The figure shows three views and two pictorial views of one solid part (mm, origin at its lowest corner). Answer the questions. A direction names the side the tool comes from. Round coordinates to 2 decimals unless told otherwise and drop trailing zeros. Write each loop counter-clockwise with the first axis right and the second up, starting at its lowest first coordinate (ties: lowest second). Pieces come first, ordered by that corner, then holes. Notation, with made-up numbers: (21, -7) -> (44, -7) arc R33 ccw to (44, 27) -> close; hole circle Ø2 at (41.5, 71.5). An arc over 180 degrees is marked (long way). One line per item, written item: value.
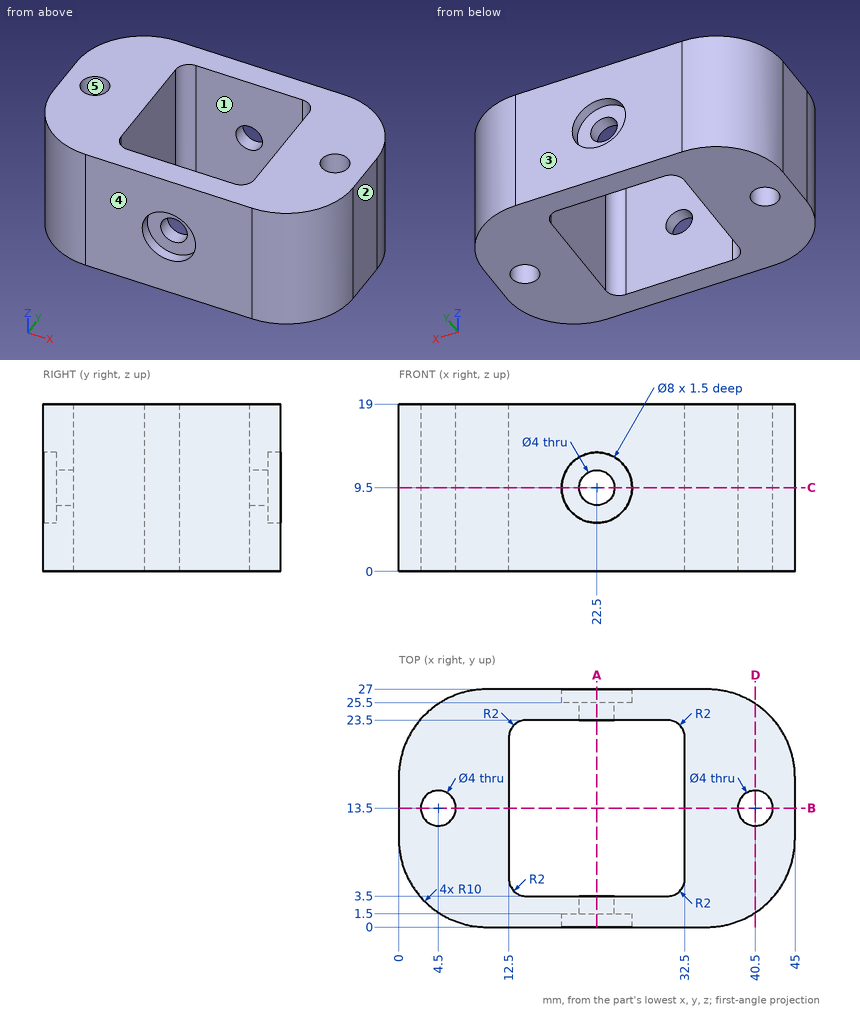
(1) Consider probe 1 along Y at (x, z) = (16, 4.75); probe 2 along Z at (x, y) = (22.5, 1.25); probe 3 along X at (y, z) = (13.75, 1.75). Determine where each line is inside the solid, lowest interval first.
Reported:
probe 1: y = 0 to 3.5, 23.5 to 27
probe 2: z = 0 to 5.5, 13.5 to 19
probe 3: x = 0 to 2.52, 6.48 to 12.5, 32.5 to 38.52, 42.48 to 45
(2) Find section B-B on y = 13.5. Give the vertices of the cut face in (x, z), plus the area to 3 significant figures.
Reported:
outline: (0, 0) -> (2.5, 0) -> (2.5, 19) -> (0, 19) -> close; (6.5, 0) -> (12.5, 0) -> (12.5, 19) -> (6.5, 19) -> close; (32.5, 0) -> (38.5, 0) -> (38.5, 19) -> (32.5, 19) -> close; (42.5, 0) -> (45, 0) -> (45, 19) -> (42.5, 19) -> close
area: 323 mm2
(3) For a pull along Y with two mould halves and no side action, classify the marked faces 3, 4 and 5 as pulls with the +Y half, pulls with the -Y half, needs draft (parallel to the pull), parting line crosses it, or undercut.
Reported:
face 3: pulls with the +Y half
face 4: pulls with the -Y half
face 5: undercut
(4) Find section D-D on x = 40.5. Give the vertices of the cut face in (y, z).
Reported:
outline: (1.65, 0) -> (11.5, 0) -> (11.5, 19) -> (1.65, 19) -> close; (15.5, 0) -> (25.35, 0) -> (25.35, 19) -> (15.5, 19) -> close
(5) Flat-ended cylindrical pins translate along their axes: pin 1 Ø2 at (x, z) = (7.5, 7.5) entering from +Y; pin 2 Ø5 at (x, z) = (22.5, 9.5) entering from -Y; pin 3 Ø2.5 at (x, y) = (40.5, 13.5) entering from -Z; pin 4 Ø6.5 at (x, z) = (22.5, 9.5) entering from +Y. Find the tip coordinate at first contact, or state that the pin passes through.
Reported:
pin 1: stops at y = 26.89
pin 2: stops at y = 1.5
pin 3: passes through
pin 4: stops at y = 25.5
(6) A tool of negligible diameter and unlimited length cuts with its end or side. For the marked faces 1 and 2, from which of +Z, -Z, +X, -X, +Y, -Y can it reach the whole face along a straight path? Write none if from no direction.
Reported:
face 1: +Z, -Z
face 2: +Z, -Z, +X, +Y, -Y
(7) Find section A-A on x = 22.5. Give the vertices of the cut face in (y, z), plus the area to 3 significant figures.
Reported:
outline: (0, 0) -> (3.5, 0) -> (3.5, 7.5) -> (1.5, 7.5) -> (1.5, 5.5) -> (0, 5.5) -> close; (0, 13.5) -> (1.5, 13.5) -> (1.5, 11.5) -> (3.5, 11.5) -> (3.5, 19) -> (0, 19) -> close; (23.5, 0) -> (27, 0) -> (27, 5.5) -> (25.5, 5.5) -> (25.5, 7.5) -> (23.5, 7.5) -> close; (23.5, 11.5) -> (25.5, 11.5) -> (25.5, 13.5) -> (27, 13.5) -> (27, 19) -> (23.5, 19) -> close
area: 93.0 mm2
(8) Find section C-C on z = 9.5. Give the number of separate pieces and of enclosed holes in the cut face, plus the area to 3 significant figures.
Reported:
separate pieces: 2
enclosed holes: 2
area: 667 mm2
